Can you work these out from the model? Positions are in its coordinate system, mm. Face numbers are marked on the shaded views. A direction names the side the tool comes from. Coordinates: 2 decimals unless noted, no trailing zeros. Order: outer loops, then holes, each group sorted by start corner. A loop starts at its lowest first (then second) coordinate and runs counter-clockwise, first axis right, second up. Notation, with made-up numbers: (27, 13) -> (85, 13) arc R23 cw to (85, 22) -> close; hole circle Ø5 at (42, 51.5). An arc over 180 degrees is marked (long way). Answer as a JSON object with one key per item and string values. Group by question number.
(1) I want a section at C-C, the plane x = 6. List the corners of the cut face in (y, z) for me (3 decimals), plus the area to 3 significant figures.
(2) I need wall thicknesses on line 1 (X direction, y = 6.25, z = 5.75); line 2 (X direction, y = 3.5, z = 3.5); line 3 (Z direction, x = 4, y = 7.75). Which ranges of each line are inside material? Lowest first, please.
(3) I want a section at A-A, the plane y = -2.5. List the corners of the cut face in (x, z) for me.
(4) I want a section at B-B, the plane z = 4.25. List the corners of the cut face in (x, y) for me (3 decimals), plus the area to 3 significant figures.
(5) If we mould it in two halves opening along X, with no side actions, what happens to the marked faces 1, 2 and 3? For each: pulls with the +X half, pulls with the -X half, needs draft (parallel to the pull), parting line crosses it, or undercut.
(6) I want a section at D-D, the plane x = 2.5. List the corners of the cut face in (y, z) for me (3 decimals).
(7) For pin 1 (2 mm diameter, centred on y = -7.5, z = 1.5, fed in from +X); pin 2 (2.5 mm diameter, centred on y = 6, z = 3.5, fed in from +X); pin 3 (1.5 mm diameter, centred on y = 6.5, z = 6.5, fed in from +X), each with a flat end and sliding along its axis, tell me the tip position at first contact or that it passes through.
(8) Which directions (+Z, -Z, +X, -X, +Y, -Y) give clear straight access to the entire face, cutting with the end or side of a thin tool? Please do the marked faces 4 and 5.
from build123d import *

# Parameters (mm, degrees)
F1_DEPTH = 12.625


with BuildPart() as f1:
    # F0 (on Front) → F1 (new body, symmetric)
    with BuildSketch(Plane.XZ):
        with BuildLine():
            Line((0, 9), (0, 0))
            Line((0, 0), (1.75, 0))
            Line((1.75, 0), (1.75, 4.487874))
            Line((1.75, 4.487874), (1.75, 8.987874))
            ThreePointArc((1.75, 8.987874), (6.237186, 8.948706), (5.75, 4.487874))
            Line((5.75, 4.487874), (7.460699, 2.422835))
            Line((7.460699, 2.422835), (8.808343, 3.539237))
            Line((8.808343, 3.539237), (7.851427, 4.694361))
            ThreePointArc((7.851427, 4.694361), (6.12928, 10.865432), (0, 9))
        make_face()
    extrude(amount=F1_DEPTH, both=True)


solid = f1.part
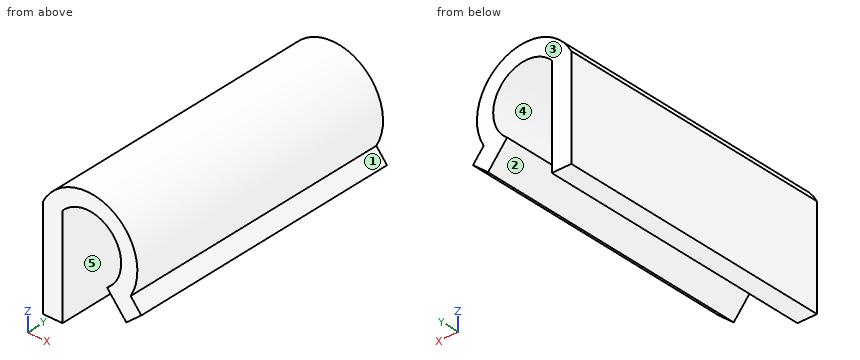
Computed values:
{
 "1": {"outline": "(-12.625, 4.186) -> (12.625, 4.186) -> (12.625, 4.69) -> (-12.625, 4.69) -> close; (-12.625, 9.187) -> (12.625, 9.187) -> (12.625, 10.934) -> (-12.625, 10.934) -> close", "area": "56.8 mm2"},
 "2": {"line 1": "x = 0 to 1.75, 6.76 to 8.29", "line 2": "x = 0 to 1.75, 6.57 to 8.76", "line 3": "z = 9.96 to 11.42"},
 "3": {"outline": "(0, 0) -> (1.75, 0) -> (1.75, 8.99) arc R3.03 cw (long way) to (5.75, 4.49) -> (7.46, 2.42) -> (8.81, 3.54) -> (7.85, 4.69) arc R4.48 ccw (long way) to (0, 9) -> close"},
 "4": {"outline": "(0, -12.625) -> (1.75, -12.625) -> (1.75, 12.625) -> (0, 12.625) -> close; (5.947, -12.625) -> (8.22, -12.625) -> (8.22, 12.625) -> (5.947, 12.625) -> close", "area": "102 mm2"},
 "5": {"face 1": "pulls with the +X half", "face 2": "undercut", "face 3": "needs draft"},
 "6": {"outline": "(-12.625, 9.58) -> (12.625, 9.58) -> (12.625, 11.167) -> (-12.625, 11.167) -> close"},
 "7": {"pin 1": "stops at x = 7.55", "pin 2": "stops at x = 8.81", "pin 3": "stops at x = 8.45"},
 "8": {"face 4": "+Y, -Y", "face 5": "-Z, +Y, -Y"}
}
